```python
from build123d import *

# Parameters (mm, degrees)
EXTRUDE_2_DEPTH        = 2
HOLE_WIZARD_M2_1_D     = 1.6
HOLE_WIZARD_M2_1_DEPTH = 5.2
HOLE_WIZARD_M2_1_TIP   = 0.480688495


with BuildPart() as part:
    # 草图2 → 凸台-拉伸2 (new body)
    with BuildSketch(Plane.XY):
        Polygon((-26.050632556, -22), (-26.050632556, -15.796671569), (-15.95719104, -3.658227581), (-0.531644656, -3.658227581), (-0.531644656, -14.822784766), (-3.721518143, -18.810126501), (-3.721518143, -22), (1.218768965, -22), (1.218768965, -20.5), (-1.781231035, -20.5), (-1.781231035, -18.4), (4.318768965, -18.4), (4.318768965, -22), (5.848102303, -22), (36.683545842, -6.316455894), (36.683545842, 0), (36.683545842, 6.316455398), (5.848102306, 22), (4.318768965, 22), (4.318768965, 18.4), (-1.781231035, 18.4), (-1.781231035, 20.5), (1.218768965, 20.5), (1.218768965, 22), (-3.721518139, 22), (-3.721518139, 18.810127986), (-0.531644652, 14.822786003), (-0.531644652, 3.65822808), (-15.95719104, 3.65822808), (-26.050632552, 15.796672063), (-26.050632552, 22), (-28.918052143, 22), (-28.918052143, 18.4), (-35.018052143, 18.4), (-35.018052143, 20.5), (-32.018052143, 20.5), (-32.018052143, 22), (-38.494101839, 22), (-38.494101839, -22), (-32.018052143, -22), (-32.018052143, -20.5), (-35.018052143, -20.5), (-35.018052143, -18.4), (-28.918052143, -18.4), (-28.918052143, -22), align=None)
        Polygon((31.367089202, 4.441746568), (30.303797872, 1.594936736), (15.417722268, 1.594936736), (15.417722268, 4.784810719), (8.86606295, 15.886233204), align=None, mode=Mode.SUBTRACT)
        Polygon((30.303797878, -1.594936257), (31.367089202, -4.441745082), (8.86606295, -15.886233452), (15.417722268, -4.784810223), (15.417722268, -1.594936257), align=None, mode=Mode.SUBTRACT)
        Polygon((5.8481023, -15.594936496), (2.658228824, -13.822784785), (2.658228824, -1.594936252), (12.227849285, -1.594936252), (12.227849285, -4.784810209), align=None, mode=Mode.SUBTRACT)
        Polygon((12.22784928, 1.594936739), (2.658228819, 1.594936739), (2.658228819, 13.822786023), (5.848102294, 15.594936248), (12.22784928, 4.784810704), align=None, mode=Mode.SUBTRACT)
        Polygon((-17.475034956, -1.79e-07), (-29.240506549, -14.620253036), (-33.493669867, -14.620253036), (-33.493669867, 14.620254005), (-29.240506547, 14.620254005), align=None, mode=Mode.SUBTRACT)
    extrude(amount=EXTRUDE_2_DEPTH)

    # M2 螺纹孔1
    with Locations(Plane.XY.offset(2)):
        with Locations((-36.994101839, 10), (-36.994101839, -10), (34.183545842, 0)):
            Hole(HOLE_WIZARD_M2_1_D / 2, depth=HOLE_WIZARD_M2_1_DEPTH)
            with Locations((0, 0, -(HOLE_WIZARD_M2_1_DEPTH + HOLE_WIZARD_M2_1_TIP / 2))):  # 118° drill point
                Cone(0, HOLE_WIZARD_M2_1_D / 2, HOLE_WIZARD_M2_1_TIP, mode=Mode.SUBTRACT)


solid = part.part
```
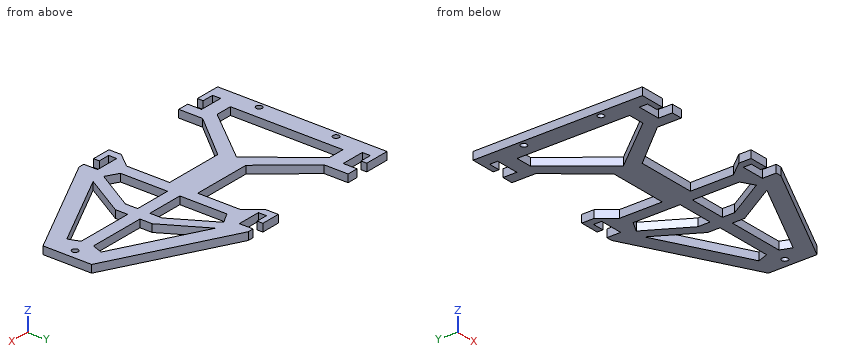
Source: CAD feature listing. Evaluate the final solid. Frame: model axes, mm. Coordinates: 2 decimals unless noted, no trailing zeros. Order: outer loops, then holes, each group sorted by start corner. A loop starts at its lowest first (then second) coordinate and runs counter-clockwise, first axis right, second up. Notation, with made-up numbers: M 46.25,69 L 96.25,69 A28 ccw 96.25,99 Z; hole C -19,-26 d10. An arc over 180 degrees is marked long. Write each question's results on one line, items separated by ' | '. Start each with the question number.
1) Line query: line 1 (Y direction, x = -33, z = 0.1); line 2 (Y direction, x = 18.5, z = 1.8); line 3 (X direction, y = -5.5, z = 1.6). Output: solid intervals per line, ascending. Write a range as from..to.
2) Section query A-A (y = 2.5). Return the cut outline in (x, z).
3) Section query B-B (x = 28). Return the cut outline in (y, z), plus the area to 3 significant figures.
4) Section query C-C (y = -10). Return the cut outline in (x, z).
5) Section query D-D (z = 1.7). Give the number of separate pieces and of enclosed holes in the cut face, plus the area to 3 significant figures.
6) Contact query for flat-ended pins moving along their axis: pin 1 Ø1 at (y, z) = (-9, 1) entering from +X; pin 2 Ø0.6 at (y, z) = (20, 0.5) entering from +X. Output: stop coordinate, or through.
Answers:
1) line 1: y = -22..-20.5, -18.4..-14.62, 14.62..18.4, 20.5..22 | line 2: y = -15.56..-10.99, -1.59..1.59, 10.99..15.56 | line 3: x = -38.49..-33.49, -21.9..-17.49, -0.53..2.66, 11.81..15, 29.29..36.68
2) outline: M -38.49,0 L -33.49,0 L -33.49,2 L -38.49,2 Z; M -19.49,0 L 2.66,0 L 2.66,2 L -19.49,2 Z; M 12.23,0 L 15.42,0 L 15.42,2 L 12.23,2 Z; M 30.64,0 L 36.68,0 L 36.68,2 L 30.64,2 Z
3) outline: M -10.73,0 L -6.15,0 L -6.15,2 L -10.73,2 Z; M -1.59,0 L 1.59,0 L 1.59,2 L -1.59,2 Z; M 6.15,0 L 10.73,0 L 10.73,2 L 6.15,2 Z | area: 24.7 mm^2
4) outline: M -38.49,0 L -37.79,0 L -37.79,2 L -38.49,2 Z; M -36.19,0 L -33.49,0 L -33.49,2 L -36.19,2 Z; M -25.52,0 L -21.23,0 L -21.23,2 L -25.52,2 Z; M -0.53,0 L 2.66,0 L 2.66,2 L -0.53,2 Z; M 9.15,0 L 12.34,0 L 12.34,2 L 9.15,2 Z; M 20.44,0 L 29.44,0 L 29.44,2 L 20.44,2 Z
5) separate pieces: 1 | enclosed holes: 8 | area: 1,210 mm^2
6) pin 1: stops at x = 32.39 | pin 2: stops at x = 10.37
